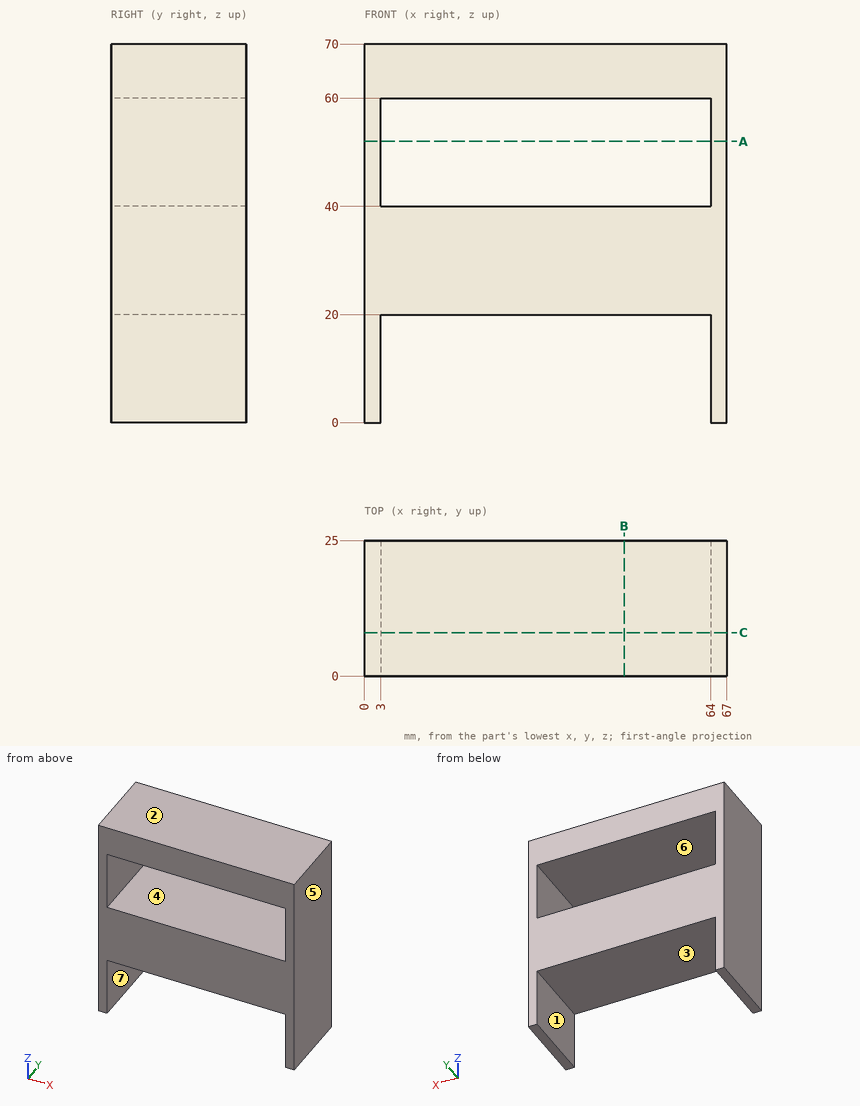
Study the drawing (mm; zero at the part's minimum x, y, z) and answer. A direction names the side the tool comes from. Coordinates: 2 decimals unless noted, no trailing zeros. Order: outer loops, then holes, each group sorted by start corner. A loop starts at its lowest first (then second) coordinate and runs counter-clockwise, first axis right, second up. Notation, with made-up numbers: M -1,88.5 L 10,88.5 A35 ccw 10,124.5 Z; hole C 38,72.5 d7. An arc over 180 degrees is marked long. Use CSV: the item, a comma, the result in double quotes.
Q1. Section A-A (z = 52) is taken. Determine the outline of the cut face in (x, y).
Here are the results:
outline,"M 0,0 L 3,0 L 3,25 L 0,25 Z; M 64,0 L 67,0 L 67,25 L 64,25 Z"
Q2. Determine the mould class of the marked faces 1, 2, 3 and 4 for opening direction Z: pulls with the +Z half, pulls with the -Z half, needs draft (parallel to the pull), parting line crosses it, or undercut.
Here are the results:
face 1,"needs draft"
face 2,"pulls with the +Z half"
face 3,"pulls with the -Z half"
face 4,"undercut"
Q3. Section C-C (y = 8) is taken. Determine the outline of the cut face in (x, z).
Here are the results:
outline,"M 0,0 L 3,0 L 3,20 L 64,20 L 64,0 L 67,0 L 67,70 L 0,70 Z; hole M 3,40 L 64,40 L 64,60 L 3,60 Z"
Q4. Section B-B (x = 48) is taken. Determine the outline of the cut face in (y, z), then the cut area to 3 significant figures.
Here are the results:
outline,"M 0,20 L 25,20 L 25,40 L 0,40 Z; M 0,60 L 25,60 L 25,70 L 0,70 Z"
area,"750 mm2"
Q5. Straight lines are drawn through the part: L1, parallel to Z at x = 42, y = 11.25; L2, parallel to X at y = 10, z = 59. For each, find the intervals that lie inside material, in ascending order.
Here are the results:
L1,"20 to 40, 60 to 70"
L2,"0 to 3, 64 to 67"
Q6. Given pin 1 Ø1.5 at (x, y) = (43.5, 3) entering from -Z, flat-ended and moving along its own axis, determine where the tip first touches the part or whether it passes through.
Here are the results:
pin 1,"z = 20"
Q7. A tool of negligible diameter and unlimited length cuts with its end or side. For the marked faces 5, 6 and 7, from which of +Z, -Z, +X, -X, +Y, -Y can it reach the whole face along a straight path? Write none if from no direction.
Here are the results:
face 5,"+Z, -Z, +X, +Y, -Y"
face 6,"+Y, -Y"
face 7,"-Z, +Y, -Y"
